```python
from build123d import *
from OCP.BRepFilletAPI import BRepFilletAPI_MakeChamfer

# Parameters (mm, degrees)
SZKIC1_W                    = 47
SZKIC1_H                    = 33
SZKIC1_R                    = 7.6
DODANIE_WYCI_GNI_CIE1_DEPTH = 5
SZKIC2_W                    = 7
SZKIC2_H                    = 20.6
DODANIE_WYCI_GNI_CIE2_DEPTH = 10
SFAZOWANIE1_SIZE            = 5
SFAZOWANIE1_SIZE2           = 2.886751346
SZKIC3_R                    = 2
WYTNIJ_WYCI_GNI_CIE1_DEPTH  = 46.131917752
ZAOKR_GLENIE1_R             = 1
DODANIE_WYCI_GNI_CIE4_START = 3
SZKIC5_W                    = 20.6
SZKIC5_H                    = 20.6
DODANIE_WYCI_GNI_CIE4_DEPTH = 3


with BuildPart() as part:
    # Szkic1 → Dodanie-wyciągnięcie1 (new body)
    # profile 1 of 3: a face of its own
    with BuildSketch(Plane.XY):
        Rectangle(SZKIC1_W, SZKIC1_H)
        Circle(SZKIC1_R, mode=Mode.SUBTRACT)
    # profile 2 of 3: a face of its own
    with BuildSketch(Plane.XY):
        with BuildLine():
            Line((4.175823272, -6.35), (-4.175823272, -6.35))
            ThreePointArc((-4.175823272, -6.35), (0, -7.6), (4.175823272, -6.35))
        make_face()
    # profile 3 of 3: a face of its own
    with BuildSketch(Plane.XY):
        with BuildLine():
            ThreePointArc((4.175823272, 6.35), (0, 7.6), (-4.175823272, 6.35))
            Line((-4.175823272, 6.35), (4.175823272, 6.35))
        make_face()
    extrude(amount=DODANIE_WYCI_GNI_CIE1_DEPTH)

    # Szkic2 → Dodanie-wyciągnięcie2 (add)
    with BuildSketch(Plane(origin=(0, 0, 0), x_dir=(-1, 0, 0), z_dir=(0, 0, -1))):
        with Locations((-13.8, 0)):
            Rectangle(SZKIC2_W, SZKIC2_H)
        with Locations((13.8, 0)):
            Rectangle(SZKIC2_W, SZKIC2_H)
    extrude(amount=DODANIE_WYCI_GNI_CIE2_DEPTH)

    # Sfazowanie1: one chamfer whose edges measure the first distance from different faces: ONE call of the kernel's chamfer builder (chamfer() names one face for all edges)
    sfazowanie1_edges_1 = [part.edges().sort_by_distance(p)[0] for p in [
        (13.8, 10.3, -10),
    ]]
    sfazowanie1_side_1 = [part.faces().sort_by_distance(p)[0] for p in [
        (13.8, 10.3, -5),
    ]]
    sfazowanie1_edges_2 = [part.edges().sort_by_distance(p)[0] for p in [
        (13.8, -10.3, -10),
    ]]
    sfazowanie1_side_2 = [part.faces().sort_by_distance(p)[0] for p in [
        (13.8, -10.3, -5),
    ]]
    sfazowanie1_edges_3 = [part.edges().sort_by_distance(p)[0] for p in [
        (-13.8, 10.3, -10),
    ]]
    sfazowanie1_side_3 = [part.faces().sort_by_distance(p)[0] for p in [
        (-13.8, 10.3, -5),
    ]]
    sfazowanie1_edges_4 = [part.edges().sort_by_distance(p)[0] for p in [
        (-13.8, -10.3, -10),
    ]]
    sfazowanie1_side_4 = [part.faces().sort_by_distance(p)[0] for p in [
        (-13.8, -10.3, -5),
    ]]
    sfazowanie1 = BRepFilletAPI_MakeChamfer(part.part.solid().wrapped)
    for e in sfazowanie1_edges_1:
        sfazowanie1.Add(SFAZOWANIE1_SIZE, SFAZOWANIE1_SIZE2, e.wrapped, sfazowanie1_side_1[0].wrapped)  # the first distance lies on this face
    for e in sfazowanie1_edges_2:
        sfazowanie1.Add(SFAZOWANIE1_SIZE, SFAZOWANIE1_SIZE2, e.wrapped, sfazowanie1_side_2[0].wrapped)  # the first distance lies on this face
    for e in sfazowanie1_edges_3:
        sfazowanie1.Add(SFAZOWANIE1_SIZE, SFAZOWANIE1_SIZE2, e.wrapped, sfazowanie1_side_3[0].wrapped)  # the first distance lies on this face
    for e in sfazowanie1_edges_4:
        sfazowanie1.Add(SFAZOWANIE1_SIZE, SFAZOWANIE1_SIZE2, e.wrapped, sfazowanie1_side_4[0].wrapped)  # the first distance lies on this face
    add(Compound.cast(sfazowanie1.Shape()), mode=Mode.REPLACE)

    # Szkic3 → Wytnij-wyciągnięcie1 (cut, through all)
    with BuildSketch(Plane(origin=(17.3, 0, 0), x_dir=(0, 0, -1), z_dir=(1, 0, 0))):
        with Locations((5, 4.3)):
            Circle(SZKIC3_R)
        with Locations((5, -4.3)):
            Circle(SZKIC3_R)
    extrude(amount=-WYTNIJ_WYCI_GNI_CIE1_DEPTH, mode=Mode.SUBTRACT)

    # Zaokrąglenie1
    zaokr_glenie1_edges = [part.edges().sort_by_distance(p)[0] for p in [
        (-23.5, -16.5, 2.5),
        (-23.5, 16.5, 2.5),
        (23.5, 16.5, 2.5),
        (23.5, -16.5, 2.5),
    ]]
    fillet(zaokr_glenie1_edges, radius=ZAOKR_GLENIE1_R)

    # Szkic5 → Dodanie-wyciągnięcie4 (add)
    with BuildSketch(Plane(origin=(0, 0, 0), x_dir=(-1, 0, 0), z_dir=(0, 0, -1)).offset(DODANIE_WYCI_GNI_CIE4_START)):
        Rectangle(SZKIC5_W, SZKIC5_H)
        with BuildLine():
            Line((4.175823272, -6.35), (-4.175823272, -6.35))
            ThreePointArc((-4.175823272, -6.35), (-7.6, 0), (-4.175823272, 6.35))
            Line((-4.175823272, 6.35), (4.175823272, 6.35))
            ThreePointArc((4.175823272, 6.35), (7.6, 0), (4.175823272, -6.35))
        make_face(mode=Mode.SUBTRACT)
    extrude(amount=-DODANIE_WYCI_GNI_CIE4_DEPTH)


solid = part.part
```
CAD build for the part. Positions are in the model's coordinates, mm. A direction names the side the tool comes from. Coordinates: 2 decimals unless noted, no trailing zeros. Write each loop counter-clockwise with the first axis right and the second up, starting at its lowest first coordinate (ties: lowest second). Pieces come first, ordered by that corner, then holes.
(1) Cut at C-C, the plane x = -16. List the corners of the cut face in (y, z), and give its area (3 significant figures).
(2) Cut at D-D, the plane y = 5.5. List the corners of the cut face in (x, z) (3 decimals), and give its area (3 significant figures).
(3) Two-plate mould, pull along Z, no slides. Class faces 3 (the face through (-13.751, 4.388, -3.002)), 4 (the face through (0, 8, 5)), 5 (the face through (0, 6.35, 1)): +Z half, -Z half, draft (parallel to the pull), parting line (faces both ways), or undercut.
(4) Cut at B-B, the plane z = 2. List the corners of the cut face in (x, y).
(5) Drill centre lines: probe 1 along Y at (x, z) = (-11, -4.75); probe 2 along Z at (x, y) = (7, -5.5); probe 3 along Z at (x, y) = (7.5, 14.5). Where is each one in solid material? Low to high.
(6) 3-axis set-ups, long thin cutter, end or side, ignore diameter. For faces 1 (the face through (-23.215, 16.199, 2.535)), 2 (the face through (0, -7, -3)): which of +Z, -Z, +X, -X, +Y, -Y reach the whole face in a straight line?
(7) Flat gauge pins, fed straight in: pin 1 (7.5 mm diameter, centred on y = -1.5, z = -8, fed in from +X); pin 2 (1.5 mm diameter, centred on x = -3.5, z = -1.5, fed in from +Y); pin 3 (7.5 mm diameter, centred on y = -3.5, z = -7, fed in from -X). Where does each tip first touch, or does it go through?
(8) Cut at A-A, the plane x = 1. List the corners of the cut face in (y, z), and give its area (3 significant figures).
Geometry says:
1. outline: (-16.5, 0) - (-10.3, 0) - (-10.3, -5) - (-7.41, -10) - (7.41, -10) - (10.3, -5) - (10.3, 0) - (16.5, 0) - (16.5, 5) - (-16.5, 5) - close; hole circle Ø4 at (-4.3, -5); hole circle Ø4 at (4.3, -5)
1. area: 331 mm2
2. outline: (-23.5, 0) - (-17.3, 0) - (-17.3, -3.4) - (-10.3, -3.4) - (-10.3, -3) - (-5.245, -3) - (-5.245, 5) - (-23.5, 5) - close; (-17.3, -10) - (-10.3, -10) - (-10.3, -6.6) - (-17.3, -6.6) - close; (5.245, -3) - (10.3, -3) - (10.3, -3.4) - (17.3, -3.4) - (17.3, 0) - (23.5, 0) - (23.5, 5) - (5.245, 5) - close; (10.3, -10) - (17.3, -10) - (17.3, -6.6) - (10.3, -6.6) - close
2. area: 308 mm2
3. face 3: undercut
3. face 4: +Z half
3. face 5: draft
4. outline: (-23.5, -15.5) arc R1 ccw to (-22.5, -16.5) - (22.5, -16.5) arc R1 ccw to (23.5, -15.5) - (23.5, 15.5) arc R1 ccw to (22.5, 16.5) - (-22.5, 16.5) arc R1 ccw to (-23.5, 15.5) - close; hole (-4.18, -6.35) - (4.18, -6.35) arc R7.6 ccw to (4.18, 6.35) - (-4.18, 6.35) arc R7.6 ccw to start
5. probe 1: y = -10.3 to -6.28, -2.32 to 2.32, 6.28 to 10.3
5. probe 2: z = -3 to 5
5. probe 3: z = 0 to 5
6. face 1: +Z, -Z, -X, +Y
6. face 2: -Z, +Y, -Y
7. pin 1: stops at x = 17.3
7. pin 2: stops at y = 10.3
7. pin 3: stops at x = -17.3
8. outline: (-16.5, 0) - (-10.3, 0) - (-10.3, -3) - (-6.35, -3) - (-6.35, 5) - (-16.5, 5) - close; (6.35, -3) - (10.3, -3) - (10.3, 0) - (16.5, 0) - (16.5, 5) - (6.35, 5) - close
8. area: 125 mm2
